Can you work these out from the model? Positions are in its coordinate system, mm. Coordinates: 2 decimals unless noted, no trailing zeros. Loops run counter-clockwise (first coordinate to the right, second up) from the corner with the lowest first, then second, coordinate; pieces in that order, holes last. Notation, with made-up numbers: (71.25, 44.5) - (83.25, 44.5) arc R18 cw to (83.25, 68.5) - close; hole circle Ø5 at (89.5, 12). An arc over 180 degrees is marked (long way). Put each result on its own line as item: value. Start each with the question number.
from build123d import *

# Parameters (mm, degrees)
SKETCH_1_W          = 69.8
SKETCH_1_H          = 49.8
EXTRUDE_1_DEPTH     = 2.4
SKETCH_2_R          = 1.5
SKETCH_2_R_2        = 5.05
CUT_EXTRUDE_3_DEPTH = 10
FILLET_4_R          = 10
FILLET_5_R          = 10


with BuildPart() as part:
    # 草图1 → 凸台-拉伸1 (new body)
    with BuildSketch(Plane.XY):
        Rectangle(SKETCH_1_W, SKETCH_1_H)
    extrude(amount=EXTRUDE_1_DEPTH)

    # 草图2 → 切除-拉伸3 (cut)
    # profile 1 of 35: a face of its own
    with BuildSketch(Plane.XY.offset(2.4)):
        with Locations((30, 20)):
            Circle(SKETCH_2_R)
    # profile 2 of 35: a face of its own
    with BuildSketch(Plane.XY.offset(2.4)):
        with Locations((20, 20)):
            Circle(SKETCH_2_R)
    # profile 3 of 35: a face of its own
    with BuildSketch(Plane.XY.offset(2.4)):
        with Locations((10, 20)):
            Circle(SKETCH_2_R)
    # profile 4 of 35: a face of its own
    with BuildSketch(Plane.XY.offset(2.4)):
        with Locations((0, 20)):
            Circle(SKETCH_2_R)
    # profile 5 of 35: a face of its own
    with BuildSketch(Plane.XY.offset(2.4)):
        with Locations((-10, 20)):
            Circle(SKETCH_2_R)
    # profile 6 of 35: a face of its own
    with BuildSketch(Plane.XY.offset(2.4)):
        with Locations((-20, 20)):
            Circle(SKETCH_2_R)
    # profile 7 of 35: a face of its own
    with BuildSketch(Plane.XY.offset(2.4)):
        with Locations((-30, 20)):
            Circle(SKETCH_2_R)
    # profile 8 of 35: a face of its own
    with BuildSketch(Plane.XY.offset(2.4)):
        with Locations((20, 10)):
            Circle(SKETCH_2_R)
    # profile 9 of 35: a face of its own
    with BuildSketch(Plane.XY.offset(2.4)):
        with Locations((10, 10)):
            Circle(SKETCH_2_R)
    # profile 10 of 35: a face of its own
    with BuildSketch(Plane.XY.offset(2.4)):
        with Locations((0, 10)):
            Circle(SKETCH_2_R)
    # profile 11 of 35: a face of its own
    with BuildSketch(Plane.XY.offset(2.4)):
        with Locations((-10, 10)):
            Circle(SKETCH_2_R)
    # profile 12 of 35: a face of its own
    with BuildSketch(Plane.XY.offset(2.4)):
        with Locations((-20, 10)):
            Circle(SKETCH_2_R)
    # profile 13 of 35: a face of its own
    with BuildSketch(Plane.XY.offset(2.4)):
        with Locations((-30, 10)):
            Circle(SKETCH_2_R)
    # profile 14 of 35: a face of its own
    with BuildSketch(Plane.XY.offset(2.4)):
        with Locations((10, 0)):
            Circle(SKETCH_2_R)
    # profile 15 of 35: a face of its own
    with BuildSketch(Plane.XY.offset(2.4)):
        Circle(SKETCH_2_R)
    # profile 16 of 35: a face of its own
    with BuildSketch(Plane.XY.offset(2.4)):
        with Locations((-10, 0)):
            Circle(SKETCH_2_R)
    # profile 17 of 35: a face of its own
    with BuildSketch(Plane.XY.offset(2.4)):
        with Locations((-30, 0)):
            Circle(SKETCH_2_R)
    # profile 18 of 35: a face of its own
    with BuildSketch(Plane.XY.offset(2.4)):
        with Locations((20, -10)):
            Circle(SKETCH_2_R)
    # profile 19 of 35: a face of its own
    with BuildSketch(Plane.XY.offset(2.4)):
        with Locations((10, -10)):
            Circle(SKETCH_2_R)
    # profile 20 of 35: a face of its own
    with BuildSketch(Plane.XY.offset(2.4)):
        with Locations((0, -10)):
            Circle(SKETCH_2_R)
    # profile 21 of 35: a face of its own
    with BuildSketch(Plane.XY.offset(2.4)):
        with Locations((-10, -10)):
            Circle(SKETCH_2_R)
    # profile 22 of 35: a face of its own
    with BuildSketch(Plane.XY.offset(2.4)):
        with Locations((-20, -10)):
            Circle(SKETCH_2_R)
    # profile 23 of 35: a face of its own
    with BuildSketch(Plane.XY.offset(2.4)):
        with Locations((-30, -10)):
            Circle(SKETCH_2_R)
    # profile 24 of 35: a face of its own
    with BuildSketch(Plane.XY.offset(2.4)):
        with Locations((20, -20)):
            Circle(SKETCH_2_R)
    # profile 25 of 35: a face of its own
    with BuildSketch(Plane.XY.offset(2.4)):
        with Locations((10, -20)):
            Circle(SKETCH_2_R)
    # profile 26 of 35: a face of its own
    with BuildSketch(Plane.XY.offset(2.4)):
        with Locations((0, -20)):
            Circle(SKETCH_2_R)
    # profile 27 of 35: a face of its own
    with BuildSketch(Plane.XY.offset(2.4)):
        with Locations((-10, -20)):
            Circle(SKETCH_2_R)
    # profile 28 of 35: a face of its own
    with BuildSketch(Plane.XY.offset(2.4)):
        with Locations((-20, -20)):
            Circle(SKETCH_2_R)
    # profile 29 of 35: a face of its own
    with BuildSketch(Plane.XY.offset(2.4)):
        with Locations((-30, -20)):
            Circle(SKETCH_2_R)
    # profile 30 of 35: a face of its own
    with BuildSketch(Plane.XY.offset(2.4)):
        with Locations((30, 10)):
            Circle(SKETCH_2_R)
    # profile 31 of 35: a face of its own
    with BuildSketch(Plane.XY.offset(2.4)):
        with Locations((30, 0)):
            Circle(SKETCH_2_R)
    # profile 32 of 35: a face of its own
    with BuildSketch(Plane.XY.offset(2.4)):
        with Locations((30, -10)):
            Circle(SKETCH_2_R)
    # profile 33 of 35: a face of its own
    with BuildSketch(Plane.XY.offset(2.4)):
        with Locations((30, -20)):
            Circle(SKETCH_2_R)
    # profile 34 of 35: a face of its own
    with BuildSketch(Plane.XY.offset(2.4)):
        with Locations((-20, 0)):
            Circle(SKETCH_2_R_2)
        with Locations((-20, 0)):
            Circle(SKETCH_2_R, mode=Mode.SUBTRACT)
    # profile 35 of 35: a face of its own
    with BuildSketch(Plane.XY.offset(2.4)):
        with Locations((20, 0)):
            Circle(SKETCH_2_R_2)
        with Locations((20, 0)):
            Circle(SKETCH_2_R, mode=Mode.SUBTRACT)
    extrude(amount=-CUT_EXTRUDE_3_DEPTH, mode=Mode.SUBTRACT)


with BuildPart() as cut_extrude_3_kept_piece:
    # of the separate pieces the step leaves, the one the design keeps (cut_extrude_3_pieces_kept)
    add(part.part.solids().sort_by_distance((34.9, -24.9, 0))[0])

    # 圆角4
    fillet_4_edges = [cut_extrude_3_kept_piece.edges().sort_by_distance(p)[0] for p in [
        (34.9, 24.9, 1.2),
    ]]
    fillet(fillet_4_edges, radius=FILLET_4_R)

    # 圆角5
    fillet_5_edges = [cut_extrude_3_kept_piece.edges().sort_by_distance(p)[0] for p in [
        (-34.9, 24.9, 1.2),
        (-34.9, -24.9, 1.2),
        (34.9, -24.9, 1.2),
    ]]
    fillet(fillet_5_edges, radius=FILLET_5_R)


solid = cut_extrude_3_kept_piece.part
Q1. We'd pull the mould along X, two halves only. Please class faces 1 (the cylindrical face through (28.5, 10.07, 1.22)), 2 (the cylindrical face through (8.89, -18.99, 1.22)), 3 (the flat face through (0, -24.9, 1)): released by +X, released by -X, zero draft, split by the parting line, or undercut.
Q2. I want a section at A-A on x = 20. List the corners of the cut face in (y, z) for me, and give its area (3 significant figures).
Q3. I want a section at B-B on y = -10. Count the separate pieces of the cut face and the enclosed holes in it, and give its area (3 significant figures).
Q4. I want a section at C-C on x = -23.5. List the corners of the cut face in (y, z) for me.
Q5. Will this pin go through, and if not, where does the flat tip stop? pin 1 (8 mm diameter, centred on x = 20, y = 0, fed in from -Z).
Q6. Please list where these lines run through material, in increasing order: line 1 along Y through (x, z) = (-20, 0.55); line 2 along Y through (x, z) = (-10, 1.7); line 3 along X through (y, z) = (-2.5, 1.85). Write a range as [from, to].
Calculated:
1. face 1: undercut
1. face 2: undercut
1. face 3: zero draft
2. outline: (-24.9, 0) - (-21.5, 0) - (-21.5, 2.4) - (-24.9, 2.4) - close; (-18.5, 0) - (-11.5, 0) - (-11.5, 2.4) - (-18.5, 2.4) - close; (-8.5, 0) - (-5.05, 0) - (-5.05, 2.4) - (-8.5, 2.4) - close; (5.05, 0) - (8.5, 0) - (8.5, 2.4) - (5.05, 2.4) - close; (11.5, 0) - (18.5, 0) - (18.5, 2.4) - (11.5, 2.4) - close; (21.5, 0) - (24.9, 0) - (24.9, 2.4) - (21.5, 2.4) - close
2. area: 66.5 mm2
3. separate pieces: 8
3. enclosed holes: 0
3. area: 117 mm2
4. outline: (-24.9, 0) - (-3.64, 0) - (-3.64, 2.4) - (-24.9, 2.4) - close; (3.64, 0) - (24.9, 0) - (24.9, 2.4) - (3.64, 2.4) - close
5. pin 1: through
6. line 1: [-24.9, -21.5], [-18.5, -11.5], [-8.5, -5.05], [5.05, 8.5], [11.5, 18.5], [21.5, 24.9]
6. line 2: [-24.9, -21.5], [-18.5, -11.5], [-8.5, -1.5], [1.5, 8.5], [11.5, 18.5], [21.5, 24.9]
6. line 3: [-34.9, -24.39], [-15.61, 15.61], [24.39, 34.9]
